from build123d import *

# Parameters (mm, degrees)
SKETCH1_R           = 10
BOSS_EXTRUDE1_DEPTH = 21
SKETCH_1_R          = 6
EXTRUDE_1_DEPTH     = 15
FILLET_1_R          = 1


with BuildPart() as part:
    # Sketch1 → Boss-Extrude1 (new body, symmetric)
    with BuildSketch(Plane(origin=(0, 0, 0), x_dir=(0, 0, -1), z_dir=(1, 0, 0))):
        Circle(SKETCH1_R)
    extrude(amount=BOSS_EXTRUDE1_DEPTH, both=True)

    # 草图1 → 凸台-拉伸1 (add)
    with BuildSketch(Plane(origin=(21, 0, 0), x_dir=(0, 0, -1), z_dir=(1, 0, 0))):
        Circle(SKETCH_1_R)
    extrude_1 = extrude(amount=EXTRUDE_1_DEPTH)

    # 镜向1: 凸台-拉伸1 across plane
    add(extrude_1.mirror(Plane(origin=(0, 0, 0), x_dir=(0, 0, 1), z_dir=(1, 0, 0))))

    # 圆角1
    fillet_1_edges = [part.edges().sort_by_distance(p)[0] for p in [
        (-21, 0, 6),
        (21, 0, 6),
    ]]
    fillet(fillet_1_edges, radius=FILLET_1_R)


solid = part.part
Source: CAD feature listing. Evaluate the final solid. Frame: model axes, mm. A direction names the side the tool comes from. Round coordinates to 2 decimals unless told otherwise and drop trailing zeros. Loops run counter-clockwise (first coordinate to the right, second up) from the corner with the lowest first, then second, coordinate; pieces in that order, holes last. Notation, with made-up numbers: (-29.5, 2) -> (-15.5, 2) arc R17 ccw to (-15.5, 13) -> close; hole circle Ø9 at (-10.75, 48). An arc over 180 degrees is marked (long way). Answer as a JSON object with one key per item and string values. Group by question number.
Q1. Section query C-C (x = 26). Output: boundary loops of the cut face in (y, z), plus the area to 3 significant figures.
Q2. Section query D-D (x = 5). Output: boundary loops of the cut face in (y, z).
Q3. Ray query, line 1 (X direction, y = -2, z = -7); line 2 (Z direction, x = 0, y = 8); line 3 (Y direction, x = 32, z = 0.25). Return the intervals inside material, ascending. Write a range as from..to.
Q4. Access query for faces 1 (the flat face through (-21, -2, 7)), 2 (the cylindrical face through (0.29, -9.76, 2.17)), 3 (the cylindrical face through (29, 0, 6)). Directions: +Z, -Z, +X, -X, +Y, -Y. A direction counts if a zero-diameter tool reaches every point of the face in a straight line with its end or side. Return the directions, or none.
Q5. Contact query for flat-ended pins moving along their axis: P1, Ø1, axis at x = 4.5, z = 7.5, coming from the +Y side; P2, Ø2, axis at x = -0.5, z = -6, coming from the +Y side; P3, Ø3, axis at x = -22, z = -4, coming from the -Y side. Output: stop coordinate, or through.
Q6. Section query A-A (y = 0). Output: boundary loops of the cut face in (x, z), plus the area to 3 significant figures.
Completed:
{
 "1": {"outline": "circle Ø12 at (0, 0)", "area": "113 mm²"},
 "2": {"outline": "circle Ø20 at (0, 0)"},
 "3": {"line 1": "-21..21", "line 2": "-6..6", "line 3": "-5.99..5.99"},
 "4": {"face 1": "-X", "face 2": "+X, -X", "face 3": "+X"},
 "5": {"P1": "y = 7.14", "P2": "y = 8.66", "P3": "y = -9.58"},
 "6": {"outline": "(-36, -6) -> (-22, -6) arc R1 cw to (-21, -7) -> (-21, -10) -> (21, -10) -> (21, -7) arc R1 cw to (22, -6) -> (36, -6) -> (36, 6) -> (22, 6) arc R1 cw to (21, 7) -> (21, 10) -> (-21, 10) -> (-21, 7) arc R1 cw to (-22, 6) -> (-36, 6) -> close", "area": "1,200 mm²"}
}
